Geometry check sheet. Reference: the model listing, model coordinates, mm. Face numbers are marked on the shaded views. A direction names the side the tool comes from. Give positions to 0.01 mm unless a question says otherwise; leave off trailing zeros. Loops run counter-clockwise (first coordinate to the right, second up) from the corner with the lowest first, then second, coordinate; pieces in that order, holes last. Notation, with made-up numbers: (69.5, 42.25) - (87.5, 42.25) arc R38 ccw to (87.5, 81.25) - close; hole circle Ø8 at (-22, 32.5). An arc over 180 degrees is marked (long way). Use a Markdown table: item, result. Add a question column.
1. Cross-section at A-A on x = 39. Enter the section's corners in (y, z).
2. Depth check by flat-ended pin: P1, Ø3, axis at x = -40.6, z = -18, coming from the +Y side; P2, Ø4, axis at x = 39, z = 25, coming from the -Y side; P3, Ø10, axis at y = -30, z = -17.5, coming from the +X side; P4, Ø3, axis at x = 3.5, y = -15, coming from the -Z side. Enter the tip coordinate at first touch or a pass-through.
3. Cross-section at B-B on x = -40.6. Enter the section's corners in (y, z), and give its area (3 significant figures).
4. Set-up check for the marked faces 1 and 2: record each of +Z, -Z, +X, -X, +Y, -Y from which the full face is reachable in a straight line by a thin tool's end or side.
5. Material ranges on L1, parallel to X at y = -0.4, z = 0; L2, parallel to X at y = -0.2, z = 18; L3, parallel to Y at x = -41.5, z = 16, recorded low to high.
from build123d import *

# Parameters (mm, degrees)
SKETCH1_W           = 93.2
SKETCH1_H           = 83
BOSS_EXTRUDE1_DEPTH = 9.55
BOSS_EXTRUDE3_DEPTH = 2.5
SKETCH6_R           = 1.2
CUT_EXTRUDE1_DEPTH  = 0.9


with BuildPart() as part:
    # Sketch1 → Boss-Extrude1 (new body)
    with BuildSketch(Plane(origin=(0, 0, 0), x_dir=(1, 0, 0), z_dir=(0, 1, 0))):
        Rectangle(SKETCH1_W, SKETCH1_H)
    extrude(amount=-BOSS_EXTRUDE1_DEPTH)

    # Sketch3 → Loft3 section 0
    with BuildSketch(Plane(origin=(0, -35.75, 0), x_dir=(-1, 0, 0), z_dir=(0, -1, 0))):
        with BuildLine():
            Line((0.25082265, 26.712128254), (-25.912128254, 0.54917735))
            Line((-25.912128254, 0.54917735), (-25.362950904, 0))
            Line((-25.362950904, 0), (-25.912128254, -0.54917735))
            Line((-25.912128254, -0.54917735), (0.25082265, -26.712128254))
            Line((0.25082265, -26.712128254), (0.8, -26.162950904))
            Line((0.8, -26.162950904), (1.34917735, -26.712128254))
            Line((1.34917735, -26.712128254), (27.512128254, -0.54917735))
            Line((27.512128254, -0.54917735), (26.962950904, 0))
            Line((26.962950904, 0), (27.512128254, 0.54917735))
            Line((27.512128254, 0.54917735), (1.34917735, 26.712128254))
            Line((1.34917735, 26.712128254), (0.8, 26.162950904))
            Line((0.8, 26.162950904), (0.25082265, 26.712128254))
        make_face()
    # Sketch2 → Loft3 section 1
    with BuildSketch(Plane.XZ.offset(9.55)):
        with BuildLine():
            Line((-10.718342201, -38.202613448), (-0.8, -28.284271247))
            Line((-0.8, -28.284271247), (9.118342201, -38.202613448))
            Line((9.118342201, -38.202613448), (37.402613448, -9.918342201))
            Line((37.402613448, -9.918342201), (27.484271247, 0))
            Line((27.484271247, 0), (37.402613448, 9.918342201))
            Line((37.402613448, 9.918342201), (9.118342201, 38.202613448))
            Line((9.118342201, 38.202613448), (-0.8, 28.284271247))
            Line((-0.8, 28.284271247), (-10.718342201, 38.202613448))
            Line((-10.718342201, 38.202613448), (-39.002613448, 9.918342201))
            Line((-39.002613448, 9.918342201), (-29.084271247, 0))
            Line((-29.084271247, 0), (-39.002613448, -9.918342201))
            Line((-39.002613448, -9.918342201), (-10.718342201, -38.202613448))
        make_face()
    loft()

    # Sketch5 → Boss-Extrude3 (add)
    with BuildSketch(Plane.XZ.offset(35.75)):
        Polygon((-0.8, -26.162950904), (-0.25082265, -26.712128254), (25.912128254, -0.54917735), (25.362950904, 0), (25.912128254, 0.54917735), (-0.25082265, 26.712128254), (-0.8, 26.162950904), (-1.34917735, 26.712128254), (-27.512128254, 0.54917735), (-26.962950904, 0), (-27.512128254, -0.54917735), (-1.34917735, -26.712128254), align=None)
    extrude(amount=BOSS_EXTRUDE3_DEPTH)

    # Sketch6 → Cut-Extrude1 (cut)
    with BuildSketch(Plane(origin=(0, 0, 0), x_dir=(1, 0, 0), z_dir=(0, 1, 0))):
        with Locations(Location((39, -25, 0), (0, 0, 270))):
            Circle(SKETCH6_R)
        with Locations(Location((39, 0, 0), (0, 0, 270))):
            Circle(SKETCH6_R)
        with Locations(Location((39, 25, 0), (0, 0, 270))):
            Circle(SKETCH6_R)
        with Locations(Location((-40.6, 18, 0), (0, 0, 270))):
            Circle(SKETCH6_R)
        with Locations(Location((-40.6, -18, 0), (0, 0, 270))):
            Circle(SKETCH6_R)
        with Locations(Location((-0.8, -25, 0), (0, 0, 270))):
            Circle(SKETCH6_R)
        with Locations(Location((-0.8, 0, 0), (0, 0, 270))):
            Circle(SKETCH6_R)
        with Locations(Location((-0.8, 25, 0), (0, 0, 270))):
            Circle(SKETCH6_R)
    extrude(amount=-CUT_EXTRUDE1_DEPTH, mode=Mode.SUBTRACT)


solid = part.part
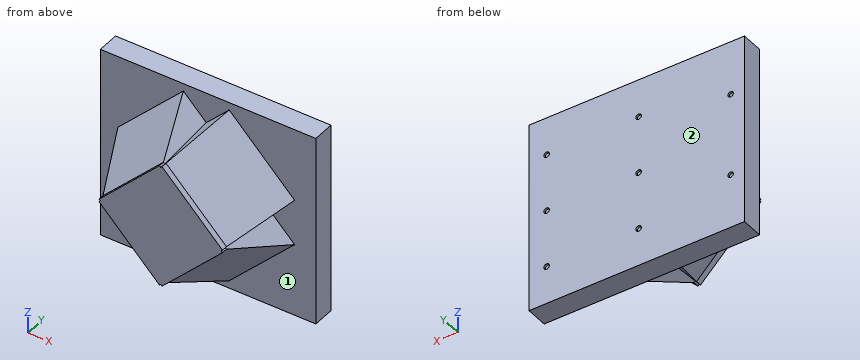
Values found:
| question | item | result |
|---|---|---|
| 1 | outline | (-9.55, -41.5) - (0, -41.5) - (0, -26.2) - (-0.9, -26.2) - (-0.9, -23.8) - (0, -23.8) - (0, -1.2) - (-0.9, -1.2) - (-0.9, 1.2) - (0, 1.2) - (0, 23.8) - (-0.9, 23.8) - (-0.9, 26.2) - (0, 26.2) - (0, 41.5) - (-9.55, 41.5) - close |
| 2 | P1 | stops at y = 0 |
| 2 | P2 | stops at y = -9.55 |
| 2 | P3 | stops at x = 19.93 |
| 2 | P4 | stops at z = -33.65 |
| 3 | outline | (-9.55, -41.5) - (0, -41.5) - (0, -19.2) - (-0.9, -19.2) - (-0.9, -16.8) - (0, -16.8) - (0, 16.8) - (-0.9, 16.8) - (-0.9, 19.2) - (0, 19.2) - (0, 41.5) - (-9.55, 41.5) - close |
| 3 | area | 788 mm2 |
| 4 | face 1 | -Y |
| 4 | face 2 | +Z, -Z, +X, -X, +Y |
| 5 | L1 | x = -46.6 to -2, 0.4 to 37.8, 40.2 to 46.6 |
| 5 | L2 | x = -46.6 to -41.8, -39.4 to 46.6 |
| 5 | L3 | y = -9.55 to 0 |
